from build123d import *

# Parameters (mm, degrees)
F1_DEPTH  = 5
F2_W      = 7
F2_H      = 2.1077826433
F2_W_2    = 1.5
F2_H_2    = 2.502781529
F2_H_3    = 3.0992894471
F3_DEPTH  = 5
F4_R      = 0.5
F5_DEPTH  = 0.5
F6_R      = 0.5
F7_DEPTH  = 0.5
F8_R      = 0.5
F9_DEPTH  = 0.5
F10_R     = 0.5
F11_DEPTH = 0.5


with BuildPart() as f1:
    # F0 (on Right) → F1 (new body, symmetric)
    with BuildSketch(Plane.YZ):
        with BuildLine():
            ThreePointArc((5, -1), (6, 0), (5, 1))
            Line((5, 1), (-5, 1))
            ThreePointArc((-5, 1), (-6, 0), (-5, -1))
            Line((-5, -1), (5, -1))
        make_face()
    extrude(amount=F1_DEPTH, both=True)

    # F2 (on face) → F3 (cut)
    with BuildSketch(Plane.XY.offset(1)):
        with Locations((0, 5.0538913216)):
            Rectangle(F2_W, F2_H)
        with Locations((-4.25, -5.2513907645)):
            Rectangle(F2_W_2, F2_H_2)
        with Locations((4.25, -5.5496447235)):
            Rectangle(F2_W_2, F2_H_3)
    extrude(amount=-F3_DEPTH, mode=Mode.SUBTRACT)

    # F4 (on face) → F5 (cut)
    with BuildSketch(Plane(origin=(-3.5, 0, 0), x_dir=(0, -1, 0), z_dir=(-1, 0, 0))):
        with Locations((5, 0)):
            Circle(F4_R)
    extrude(amount=-F5_DEPTH, mode=Mode.SUBTRACT)

    # F6 (on face) → F7 (cut)
    with BuildSketch(Plane.YZ.offset(3.5)):
        with Locations((-5, 0)):
            Circle(F6_R)
    extrude(amount=-F7_DEPTH, mode=Mode.SUBTRACT)

    # F8 (on face) → F9 (join)
    with BuildSketch(Plane.YZ.offset(-3.5)):
        with Locations((5, 0)):
            Circle(F8_R)
    extrude(amount=F9_DEPTH)

    # F10 (on face) → F11 (join)
    with BuildSketch(Plane(origin=(3.5, 0, 0), x_dir=(0, -1, 0), z_dir=(-1, 0, 0))):
        with Locations((-5, 0)):
            Circle(F10_R)
    extrude(amount=F11_DEPTH)


solid = f1.part
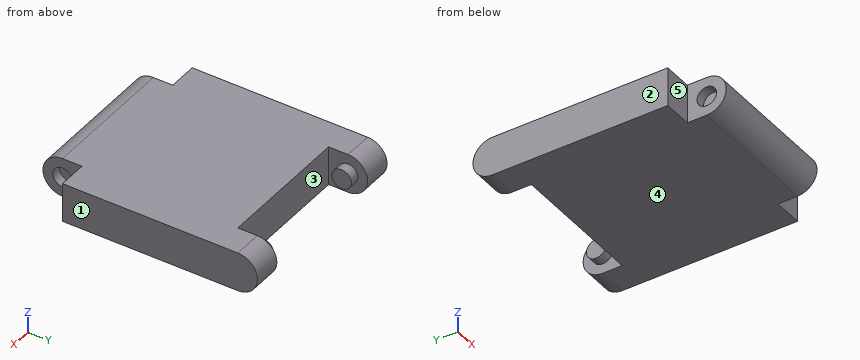
The model under review builds one solid part; all positions refer to its coordinate system, in mm. Face numbers are marked on the shaded views. A direction names the side the tool comes from. Round coordinates to 2 decimals unless told otherwise and drop trailing zeros. Loops run counter-clockwise (first coordinate to the right, second up) from the corner with the lowest first, then second, coordinate; pieces in that order, holes last. Notation, with made-up numbers: M -16.5,-0.5 L 10.5,-0.5 A5 cw 10.5,7.5 Z; hole C 51,-8.75 d10. An arc over 180 degrees is marked long. Answer as CSV lines item,"result". Start each with the question number.
Item 1: Mouldability with a two-part tool opening along X and no side actions: class the marked faces 1, 2 and 3 as released by +X, released by -X, zero draft, split by the parting line, or undercut.
Item 2: For the marked faces 4 and 5, list the 3-axis set-ups (+Z, -Z, +X, -X, +Y, -Y) from which the entire face can be reached by the end or side of a thin tool; tool diameter is ignored.
Item 3: Consider section C-C (z = -0.75). Write out the cut boundary in (x, y), then the cut area to 3 significant figures.
Item 4: Wall thickness on line 1 (X direction, y = 5, z = 0.15); line 2 (X direction, y = 4.25, z = 0.55); line 3 (Z direction, x = -3.4, y = -5): over which ranges is each line inside the solid? List them lowest first. Write a range as [from, to].
Item 5: Consider section B-B (x = 0). Write out the cut boundary in (y, z), then the cut area to 3 significant figures.
Item 6: Consider section A-A (z = 0). Write out the cut boundary in (x, y), then the cut area to 4 significant figures.
Item 7: Insertion check: P1, Ø1.2, axis at x = -4, z = 0, coming from the -Y side; P2, Ø0.8, axis at y = -5, z = 0, coming from the +X side; P3, Ø0.6, axis at x = 0.5, z = 0, coming from the +Y side. Each pin has a flat end and moves straight along its axis. Give the tip position at first contact, or say it passes through.
Answer:
1,face 1,"released by +X"
1,face 2,"released by -X"
1,face 3,"undercut"
2,face 4,"-Z, +X, -X, +Y, -Y"
2,face 5,"+Z, -Z, -X, -Y"
3,outline,"M -5,-4 L -3.5,-4 L -3.5,-5.66 L 3.5,-5.66 L 3.5,-4 L 5,-4 L 5,5.66 L 3.5,5.66 L 3.5,4 L -3.5,4 L -3.5,5.66 L -5,5.66 Z"
3,area,"96.6 mm^2"
4,line 1,"x = [-5, -3], [3, 5]"
4,line 2,"x = [-5, -3.5], [3.5, 5]"
4,line 3,"z = [-1, -0.5], [0.5, 1]"
5,outline,"M -5,-1 L 4,-1 L 4,1 L -5,1 A1 ccw Z"
5,area,"19.6 mm^2"
6,outline,"M -5,-4 L -3.5,-4 L -3.5,-4.5 L -3,-4.5 L -3,-5.5 L -3.5,-5.5 L -3.5,-6 L 3.5,-6 L 3.5,-5.5 L 3,-5.5 L 3,-4.5 L 3.5,-4.5 L 3.5,-4 L 5,-4 L 5,6 L 3.5,6 L 3.5,5.5 L 3,5.5 L 3,4.5 L 3.5,4.5 L 3.5,4 L -3.5,4 L -3.5,4.5 L -3,4.5 L -3,5.5 L -3.5,5.5 L -3.5,6 L -5,6 Z"
6,area,"100.0 mm^2"
7,P1,"stops at y = -6"
7,P2,"stops at x = 3"
7,P3,"stops at y = 4"
